Here's how the part is built. I have some questions about the finished solid (model axes, mm). Coordinates: 2 decimals unless noted, no trailing zeros. Write each loop counter-clockwise with the first axis right and the second up, starting at its lowest first coordinate (ties: lowest second). Pieces come first, ordered by that corner, then holes.
Item 1: I want a section at C-C (x = 349.5). Count the separate pieces of the cut face and the enclosed holes in it, and give its area (3 significant figures).
Item 2: I want a section at B-B (y = 191). Please give me the cut outline in (x, z), and give its area (3 significant figures).
Item 3: I want a section at A-A (x = 488). Please give me the cut outline in (y, z), and give its area (3 significant figures).
Item 4: I'm going to push flat-ended pins straight in: P1, Ø12, axis at x = 347, y = 277, coming from the -Z side; P2, Ø3.5, axis at x = 498, y = 267, coming from the -Z side; P3, Ø3.5, axis at x = 500.5, y = 267.5, coming from the +Z side. Where does each tip first touch, or does it pass through?
Item 5: Please list where these lines run through material, in increasing order: line 1 (X direction, y = 249.5, z = -615.5); line 2 (Y direction, x = 296, z = -655.5); line 3 (Z direction, x = 484, y = 201.5).
from build123d import *

# Parameters (mm, degrees)
SWEEP3_PROFILE_R    = 8
SWEEP4_PROFILE_R    = 8
SWEEP6_PROFILE_R    = 8
SKETCH80_W          = 50
SKETCH80_H          = 57.849509876
CUT_EXTRUDE1_DEPTH  = 300
SKETCH81_R          = 60
BOSS_EXTRUDE1_DEPTH = 70
FILLET1_R           = 10


with BuildPart() as part:
    # Sweep3: sweep along a curve in space
    with BuildLine() as sweep3_path:
        Line((480, 230, -590), (190, 190, -750))
        Line((480, 230, -590), (190, 250, -520))
    # Sweep3 profile (on start of the path) → Sweep3 (sweep)
    with BuildSketch(Plane(origin=(190, 250, -520), x_dir=(0.2346405331038965, 0, 0.9720822085732871), z_dir=(0.9699050900314443, -0.06689000620906493, -0.23411502173172755))):
        Circle(SWEEP3_PROFILE_R)
    sweep(path=sweep3_path.line, transition=Transition.RIGHT)

    # Sweep4: sweep along a curve in space
    with BuildLine() as sweep4_path:
        Line((480, 230, -590), (190, 500, -650))
    # Sweep4 profile (on start of the path) → Sweep4 (sweep)
    with BuildSketch(Plane(origin=(480, 230, -590), x_dir=(-0.6814185279188429, -0.7318939744313498, 0), z_dir=(-0.7236444363336271, 0.6737379234830321, -0.1497195385517849))):
        Circle(SWEEP4_PROFILE_R)
    sweep(path=sweep4_path.line)


with BuildPart() as body_2:
    # Sweep6: sweep along a curve in space
    with BuildLine() as sweep6_path:
        Line((480, 80, -590), (190, 90, -539.058512789))
        Line((480, 80, -590), (190, 60, -704.548891224))
    # Sweep6 profile (on start of the path) → Sweep6 (sweep)
    with BuildSketch(Plane(origin=(190, 60, -704.548891224), x_dir=(-0.3673752090170087, 0, 0.9300728228476033), z_dir=(0.9281653987551736, 0.0640114068107016, 0.3666217837932773))):
        Circle(SWEEP6_PROFILE_R)
    sweep(path=sweep6_path.line, transition=Transition.RIGHT)


with BuildPart() as cut_extrude1_tool:
    # Sketch80 → Cut-Extrude1 (new body)
    with BuildSketch(Plane(origin=(0, 0, 0), x_dir=(1, 0, 0), z_dir=(0, 1, 0))):
        with Locations((505, 590.170010545)):
            Rectangle(SKETCH80_W, SKETCH80_H)
    extrude(amount=CUT_EXTRUDE1_DEPTH)


with BuildPart() as part_1:
    add(part.part)

    # Cut-Extrude1: cut by cut_extrude1_tool
    add(cut_extrude1_tool.part, mode=Mode.SUBTRACT)

    # Sketch81 → Boss-Extrude1 (add)
    with BuildSketch(Plane(origin=(465, 0, 0), x_dir=(0, 0, -1), z_dir=(1, 0, 0))):
        with Locations((590, 155.874728278)):
            Circle(SKETCH81_R)
        with BuildLine():
            Line((620, 235), (560, 235))
            Line((560, 235), (560, 207.836252505))
            ThreePointArc((560, 207.836252505), (590, 215.874728278), (620, 207.836252505))
            Line((620, 207.836252505), (620, 235))
        make_face()
        with BuildLine():
            ThreePointArc((620, 103.91320405), (590, 95.874728278), (560, 103.91320405))
            Line((560, 103.91320405), (560, 75))
            Line((560, 75), (620, 75))
            Line((620, 75), (620, 103.91320405))
        make_face()
    extrude(amount=BOSS_EXTRUDE1_DEPTH)

    # Fillet1
    fillet1_edges = [part_1.edges().sort_by_distance(p)[0] for p in [
        (500, 235, -620),
        (500, 103.91320405, -620),
        (500, 207.836252505, -620),
        (500, 235, -560),
        (500, 207.836252505, -560),
        (500, 103.91320405, -560),
        (500, 75, -560),
        (500, 75, -620),
    ]]
    fillet(fillet1_edges, radius=FILLET1_R)


with BuildPart() as body_2_1:
    add(body_2.part)

    # Cut-Extrude1: cut by cut_extrude1_tool
    add(cut_extrude1_tool.part, mode=Mode.SUBTRACT)


with BuildPart() as part_2:
    add(part_1.part)

    # Combine1: union body 2
    add(body_2_1.part)


with BuildPart() as part_3:
    # Body-Move/Copy1: moved
    add(part_2.part.moved(Location((0, 46, 0))))


solid = part_3.part
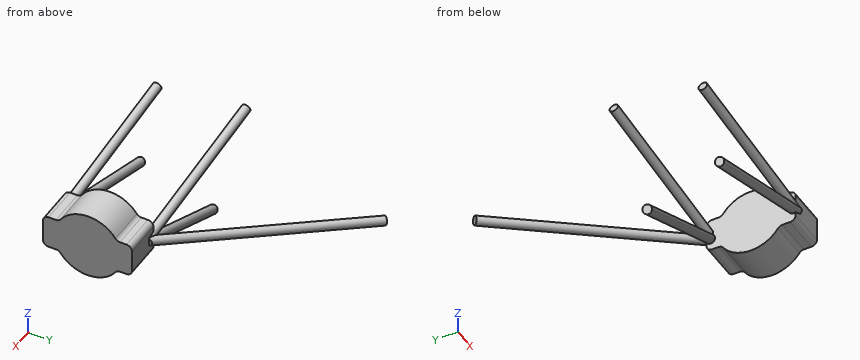
Answer:
1. separate pieces: 5
1. enclosed holes: 0
1. area: 1,140 mm2
2. outline: (465, -649.01) - (535, -649.01) - (535, -530.99) - (465, -530.99) - close
2. area: 8,260 mm2
3. outline: (121, -610) arc R10 ccw to (131, -620) - (144.43, -620) arc R10 cw to (152.64, -624.29) arc R60 ccw to (251.11, -624.29) arc R10 cw to (259.32, -620) - (271, -620) arc R10 ccw to (281, -610) - (281, -570) arc R10 ccw to (271, -560) - (259.32, -560) arc R10 cw to (251.11, -555.71) arc R60 ccw to (152.64, -555.71) arc R10 cw to (144.43, -560) - (131, -560) arc R10 ccw to (121, -570) - close
3. area: 14,000 mm2
4. P1: stops at z = -566.4
4. P2: stops at z = -620
4. P3: stops at z = -560
5. line 1: x = 465 to 535
5. line 2: y = 109.06 to 117.89
5. line 3: z = -650 to -530
